The model under review builds one solid part; all positions refer to its coordinate system, in mm. Face numbers are marked on the shaded views. A direction names the side the tool comes from. Coordinates: 2 decimals unless noted, no trailing zeros. Use one line per item in the form item = value.
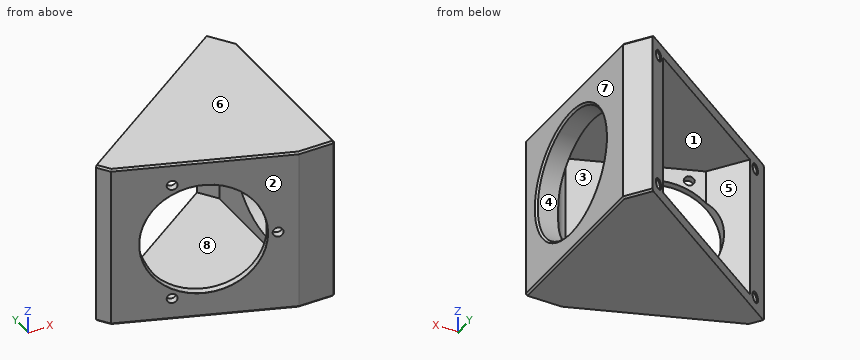
from build123d import *

# Parameters (mm, degrees)
P_IDAT_VYSUNUT_M1_DEPTH                     = 20
P_IDAT_VYSUNUT_M2_DEPTH                     = 3
V_LCOV_START                                = -141.407290306
V_LCOV_ZAHLOUBEN_PRO_M2_5_ROUBY_S_2_R       = 1.35
V_LCOV_ZAHLOUBEN_PRO_M2_5_ROUBY_S_VNI_DEPTH = 2
V_LCOV_START_2                              = -139.417290306
V_LCOV_ZAHLOUBEN_PRO_M2_5_ROUBY_S_3_O_R     = 1.4
V_LCOV_ZAHLOUBEN_PRO_M2_5_ROUBY_S_3_O_R_2   = 1.35
V_LCOV_ZAHLOUBEN_PRO_M2_5_ROUBY_S_3_DEPTH   = 0.01
SKICA13_W                                   = 63.2698
SKICA13_H                                   = 46
SKICA13_W_2                                 = 49.2698
SKICA13_H_2                                 = 40
ODEBRAT_VYSUNUT_M1_DEPTH                    = 3
M3_Z_VIT2_D                                 = 2.5
M3_Z_VIT2_DEPTH                             = 5.5
M3_Z_VIT2_CSINK_D                           = 3.05
M3_Z_VIT2_CSINK_ANGLE                       = 90
M3_Z_VIT2_TIP                               = 0.751075774
M3_Z_VIT2_ON_FACE_2_D                       = 2.5
M3_Z_VIT2_ON_FACE_2_DEPTH                   = 5.5
M3_Z_VIT2_ON_FACE_2_CSINK_D                 = 3.05
M3_Z_VIT2_ON_FACE_2_CSINK_ANGLE             = 90
M3_Z_VIT2_ON_FACE_2_TIP                     = 0.751075774
M3_Z_VIT2_ON_FACE_3_D                       = 2.5
M3_Z_VIT2_ON_FACE_3_DEPTH                   = 5.5
M3_Z_VIT2_ON_FACE_3_CSINK_D                 = 3.05
M3_Z_VIT2_ON_FACE_3_CSINK_ANGLE             = 90
M3_Z_VIT2_ON_FACE_3_TIP                     = 0.751075774
ZKOSEN_1_SIZE                               = 0.5
ZAOBLIT1_R                                  = 5


# Read off the part's stored shape, not the designer's step: Válcové zahloubení pro M2.5 šrouby s vnitřním šestihranem1
with BuildPart() as part:
    # Skica2 → Přidat vysunutím1 (new, symmetric)
    with BuildSketch(Plane.XY):
        Polygon((-340.05, -23), (-350.255276964, -23), (-394.120989631, -7.034186284), (-398.184656118, -1.23066909), (-391.631439764, 3.357942401), (-383.014556922, -8.948241654), (-350.233285651, -20.879648638), (-346.05, -20.879648638), (-346.05, 24.160174988), (-351.271982372, 31.617938704), (-346.357070106, 35.059397322), (-340.05, 26.051967722), align=None)
    extrude(amount=P_IDAT_VYSUNUT_M1_DEPTH, both=True)

    # Skica3 → Přidat vysunutím2 (add)
    with BuildSketch(Plane.XY.offset(20)):
        Polygon((-346.357070106, 35.059397322), (-340.05, 26.051967722), (-340.05, -23), (-350.255276964, -23), (-394.120989631, -7.034186284), (-398.184656118, -1.23066909), align=None)
    p_idat_vysunut_m2 = extrude(amount=P_IDAT_VYSUNUT_M2_DEPTH)

    # Zrcadlit1: Přidat vysunutím2 across plane
    add(p_idat_vysunut_m2.mirror(Plane.XY))

    # Skica6 → M36x1.0 závit1 (revolve, cut)
    with BuildSketch(Plane(origin=(-340.05, 0, 0), x_dir=(0, 0, -1), z_dir=(0, 1, 0))):
        Polygon((0, 0), (0, 6), (17.5, 6), (17.5, 0.525), (18.025, 0), align=None)
    revolve(axis=Axis((-333.7, 0, 0), (-1, 0, 0)), mode=Mode.SUBTRACT)

    # Skica8 → Ø32.0 (32) průměr díry1 (revolve, cut)
    with BuildSketch(Plane(origin=(-372.477448122, -14.911791158, 0), x_dir=(0.9396926207859314, -0.34202014332560576, 0), z_dir=(0, 0, 1))):
        Polygon((0, 0), (0, 15.613769904), (16, 6), (16, 0.025), (16.025, 0), align=None)
    revolve(axis=Axis((-374.649276032, -20.8788393, 0), (0.3420201433256057, 0.9396926207859314, 0)), mode=Mode.SUBTRACT)

    # V_lcov_ zahlouben_ pro M2.5 _rouby s 2 → Válcové zahloubení pro M2.5 šrouby s vnitřním šestihranem1 (cut)
    with BuildSketch(Plane(origin=(0, 0, 0), x_dir=(0.9396926207859079, -0.34202014332566993, 0), z_dir=(0.34202014332567, 0.939692620785908, 0)).offset(V_LCOV_START)):
        with Locations((-352.732614303, 16.76669406)):
            Circle(V_LCOV_ZAHLOUBEN_PRO_M2_5_ROUBY_S_2_R)
        with Locations((-352.732614303, -16.76669406)):
            Circle(V_LCOV_ZAHLOUBEN_PRO_M2_5_ROUBY_S_2_R)
        with Locations((-326.41417646, 0)):
            Circle(V_LCOV_ZAHLOUBEN_PRO_M2_5_ROUBY_S_2_R)
    extrude(amount=V_LCOV_ZAHLOUBEN_PRO_M2_5_ROUBY_S_VNI_DEPTH, mode=Mode.SUBTRACT)

    # V_lcov_ zahlouben_ pro M2.5 _rouby s 3 o → V_lcov_ zahlouben_ pro M2.5 _rouby s 3 (cut)
    # profile 1 of 3: a face of its own
    with BuildSketch(Plane(origin=(0, 0, 0), x_dir=(0.9396926207859079, -0.34202014332566993, 0), z_dir=(0.34202014332567, 0.939692620785908, 0)).offset(V_LCOV_START_2)):
        with Locations((-352.732614303, 16.76669406)):
            Circle(V_LCOV_ZAHLOUBEN_PRO_M2_5_ROUBY_S_3_O_R)
        with Locations((-352.732614303, 16.76669406)):
            Circle(V_LCOV_ZAHLOUBEN_PRO_M2_5_ROUBY_S_3_O_R_2, mode=Mode.SUBTRACT)
    # profile 2 of 3: a face of its own
    with BuildSketch(Plane(origin=(0, 0, 0), x_dir=(0.9396926207859079, -0.34202014332566993, 0), z_dir=(0.34202014332567, 0.939692620785908, 0)).offset(V_LCOV_START_2)):
        with Locations((-352.732614303, -16.76669406)):
            Circle(V_LCOV_ZAHLOUBEN_PRO_M2_5_ROUBY_S_3_O_R)
        with Locations((-352.732614303, -16.76669406)):
            Circle(V_LCOV_ZAHLOUBEN_PRO_M2_5_ROUBY_S_3_O_R_2, mode=Mode.SUBTRACT)
    # profile 3 of 3: a face of its own
    with BuildSketch(Plane(origin=(0, 0, 0), x_dir=(0.9396926207859079, -0.34202014332566993, 0), z_dir=(0.34202014332567, 0.939692620785908, 0)).offset(V_LCOV_START_2)):
        with Locations((-326.41417646, 0)):
            Circle(V_LCOV_ZAHLOUBEN_PRO_M2_5_ROUBY_S_3_O_R)
        with Locations((-326.41417646, 0)):
            Circle(V_LCOV_ZAHLOUBEN_PRO_M2_5_ROUBY_S_3_O_R_2, mode=Mode.SUBTRACT)
    extrude(amount=V_LCOV_ZAHLOUBEN_PRO_M2_5_ROUBY_S_3_DEPTH, mode=Mode.SUBTRACT)

    # Skica13 → Odebrat vysunutím1 (cut)
    with BuildSketch(Plane(origin=(-130.42051615, 186.259800178, 0), x_dir=(0.8191520442889952, 0.5735764363510412, 0), z_dir=(-0.5735764363510412, 0.8191520442889952, 0))):
        with Locations((-295.244757855, 0)):
            Rectangle(SKICA13_W, SKICA13_H)
        with Locations((-294.244757855, 0)):
            Rectangle(SKICA13_W_2, SKICA13_H_2, mode=Mode.SUBTRACT)
    extrude(amount=-ODEBRAT_VYSUNUT_M1_DEPTH, mode=Mode.SUBTRACT)

    # M3 závit2
    with Locations(Plane(origin=(-392.368166588, -0.820243041, 19), x_dir=(0.819152044289, 0.573576436351, 0), z_dir=(-0.573576436351, 0.819152044289, 0))):
        with Locations((0, 0)):
            CounterSinkHole(M3_Z_VIT2_D / 2, M3_Z_VIT2_CSINK_D / 2, depth=M3_Z_VIT2_DEPTH, counter_sink_angle=M3_Z_VIT2_CSINK_ANGLE)
            with Locations((0, 0, -(M3_Z_VIT2_DEPTH + M3_Z_VIT2_TIP / 2))):  # 118° drill point
                Cone(0, M3_Z_VIT2_D / 2, M3_Z_VIT2_TIP, mode=Mode.SUBTRACT)

    # M3 závit2 on face 2
    with Locations(Plane(origin=(-347.503372952, 30.594423662, -19), x_dir=(0.819152234736, 0.573576164364, 0), z_dir=(-0.573576164364, 0.819152234736, 0))):
        with Locations((0, 0), (0, -38)):
            CounterSinkHole(M3_Z_VIT2_ON_FACE_2_D / 2, M3_Z_VIT2_ON_FACE_2_CSINK_D / 2, depth=M3_Z_VIT2_ON_FACE_2_DEPTH, counter_sink_angle=M3_Z_VIT2_ON_FACE_2_CSINK_ANGLE)
            with Locations((0, 0, -(M3_Z_VIT2_ON_FACE_2_DEPTH + M3_Z_VIT2_ON_FACE_2_TIP / 2))):  # 118° drill point
                Cone(0, M3_Z_VIT2_ON_FACE_2_D / 2, M3_Z_VIT2_ON_FACE_2_TIP, mode=Mode.SUBTRACT)

    # M3 závit2 on face 3
    with Locations(Plane(origin=(-392.368166588, -0.820243041, -19), x_dir=(0.819152234736, 0.573576164364, 0), z_dir=(-0.573576164364, 0.819152234736, 0))):
        with Locations((0, 0)):
            CounterSinkHole(M3_Z_VIT2_ON_FACE_3_D / 2, M3_Z_VIT2_ON_FACE_3_CSINK_D / 2, depth=M3_Z_VIT2_ON_FACE_3_DEPTH, counter_sink_angle=M3_Z_VIT2_ON_FACE_3_CSINK_ANGLE)
            with Locations((0, 0, -(M3_Z_VIT2_ON_FACE_3_DEPTH + M3_Z_VIT2_ON_FACE_3_TIP / 2))):  # 118° drill point
                Cone(0, M3_Z_VIT2_ON_FACE_3_D / 2, M3_Z_VIT2_ON_FACE_3_TIP, mode=Mode.SUBTRACT)

    # Zkosení1
    zkosen_1_edges = [part.edges().sort_by_distance(p)[0] for p in [
        (-342.343170399, 29.326954456, -23),
        (-342.343170399, 29.326954456, 23),
        (-340.05, -23, 0),
        (-395.29245822, -5.361155754, 23),
        (-372.188133297, -15.017093142, 23),
        (-345.152638482, -23, 23),
        (-340.05, 1.525983861, 23),
        (-395.29245822, -5.361155754, -23),
        (-340.05, 1.525983861, -23),
        (-345.152638482, -23, -23),
        (-372.188133297, -15.017093142, -23),
    ]]
    chamfer(zkosen_1_edges, length=ZKOSEN_1_SIZE)

    # Zaoblit1
    # the kernel refuses this fillet: 5 mm, written as the material it adds along each edge
    with BuildSketch(Plane(origin=(-346.05, -20.879648638, 20), x_dir=(-1, 0, 0), z_dir=(0, 0, -1))) as zaoblit1_piece_1_section:
        with BuildLine():
            CenterArc((5, 4.932846812), ZAOBLIT1_R, 180, 80.599018085)
            Line((0, 4.932846812), (-0.1, 4.932846812))
            Line((-0.1, 4.932846812), (-0.1, 0))
            Line((-0.1, 0), (0, -0.1))
            ThreePointArc((0, -0.1), (2.091642826, -0.1), (4.166951364, -0.098656936))
            Line((4.166951364, -0.098656936), (4.183285651, 0))
        make_face()
    zaoblit1_piece_1 = extrude(amount=40, mode=Mode.PRIVATE)
    zaoblit1_piece_1 = zaoblit1_piece_1 - Plane(origin=(-347.091511424, 0, 0), x_dir=(0, 0, -1), z_dir=(1, 0, 0)) * Cylinder(17.5, 100, mode=Mode.PRIVATE)
    add(zaoblit1_piece_1)


solid = part.part
Item 1: To check wall thickness, follow L1, parallel to Z at x = -343, y = 0; L2, parallel to X at y = -4.5, z = -18; L3, parallel to Z at x = -363, y = 5. State the ranges of each line that lie inside material, in increasing order. Write a range as from..to.
Results found:
L1 = -23..-17.5, 17.5..23
L2 = -395.9..-390.71, -388.88..-386.13, -346.05..-340.05
L3 = -23..-20, 20..23
Item 2: Clearance check with flat-ended pins moving along their axes: pin 1 (12 mm diameter, centred on y = -2.5, z = -8.5, fed in from -X); pin 2 (10 mm diameter, centred on y = 3.5, z = -6, fed in from -X); pin 3 (8 mm diameter, centred on y = 0.5, z = 7.5, fed in from +X); pin 4 (12 mm diameter, centred on x = -368.5, z = 8.5, fed in from -Y). State where each tip first meets the part, or that it passes through.
Results found:
pin_1 = -396.46
pin_2 = -393.34
pin_3 = -386.83
pin_4 = through
Item 3: We need section A-A (z = 0). State how many separate pieces and enclosed holes the cut face has, plus the area to 3 significant figures.
Results found:
separate_pieces = 4
enclosed_holes = 0
area = 205 mm²
Item 4: Tool access review of the marked faces 1, 2, 3 and 4: name each direction out of +Z, -Z, +X, -X, +Y, -Y from which nothing blocks a thin tool from reaching the whole face with its end or side.
Results found:
face_1 = none
face_2 = +Z, -Z, -X, -Y
face_3 = +Y
face_4 = +X
Item 5: Draft analysis for pull direction Z (two halves, no side actions). For the marked faces 5, 6, 7 and 8, state which applies: released by +Z, released by -Z, zero draft, split by the parting line, or undercut.
Results found:
face_5 = undercut
face_6 = released by +Z
face_7 = zero draft
face_8 = undercut
